For this review, take the finished solid that the model builds, in its own axes (mm). Face numbers are marked on the shaded views. A direction names the side the tool comes from. Round coordinates to 2 decimals unless told otherwise and drop trailing zeros. Order: outer loops, then holes, each group sorted by start corner. A loop starts at its lowest first (then second) coordinate and runs counter-clockwise, first axis right, second up.
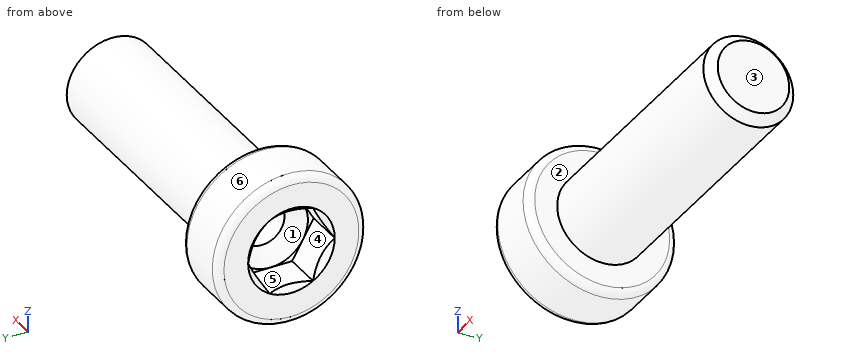
Autodesk Inventor part; units mm, degrees
ref_plane "MONTAGE_XY" through (0, 0, 0) normal (1, 0, 0) x (0, 0, -1)
ref_plane "MONTAGE_YZ" through (0, 0, 0) normal (0, 0, -1) x (0, 1, 0)
ref_plane "MONTAGE_ZX" through (0, 0, 0) normal (0, 1, 0) x (1, 0, 0)
sketch "Sketch_1" plane through (0, 0, 0) normal (0, 0, 1) x (1, 0, 0)
  line L0 (18, 0) -> (2.5, 0)
  line L1 (2.5, 0) -> (1, 1.5)
  line L2 (1, 1.5) -> (-0.5, 1.5)
  line L3 (-0.5, 1.5) -> (-1.5, 2.5)
  line L4 (-1.5, 2.5) -> (-3.6132, 2.5)
  line L5 (-3.6132, 2.5) -> (-4, 2.8868)
  line L6 (-4, 2.8868) -> (-4, 4.5)
  arc A0 (-3.5, 5) -> (-4, 4.5) centre (-3.5, 4.5) ccw
  line L7 (-3.5, 5) -> (-0.5, 5)
  arc A1 (0, 4.5) -> (-0.5, 5) centre (-0.5, 4.5) ccw
  line L8 (0, 4.5) -> (0, 3)
  line L9 (0, 3) -> (17.3865, 3)
  line L10 (17.3865, 3) -> (18, 2.3865)
  line L11 (18, 2.3865) -> (18, 0)
  line L12 (18, 0) -> (2.5, 0)
revolve "Revolution1" add sketch "Sketch_1" angle 360 about axis through (18, 0, 0) along (-1, 0, 0)
thread "Thread1"
sketch "Sketch_2" plane through (-4, 0, 0) normal (1, 0, 0) x (0, 0, -1)
  line L0 (-2.5, -1.4434) -> (0, -2.8868)
  line L1 (0, -2.8868) -> (2.5, -1.4434)
  line L2 (2.5, -1.4434) -> (2.5, 1.4434)
  line L3 (2.5, 1.4434) -> (0, 2.8868)
  line L4 (0, 2.8868) -> (-2.5, 1.4434)
  line L5 (-2.5, 1.4434) -> (-2.5, -1.4434)
extrude "Extrusion1" cut sketch "Sketch_2" along normal blind 2.5
ref_plane "MONTAGE_XY" through (0, 0, 0) normal (1, 0, 0) x (0, 0, -1)
ref_plane "MONTAGE_YZ" through (0, 0, 0) normal (0, 0, -1) x (0, 1, 0)
ref_plane "MONTAGE_ZX" through (0, 0, 0) normal (0, 1, 0) x (1, 0, 0)
ref_plane "Schrauben_punkt_XY" through (18, 0, 0) normal (-1, 0, 0) x (0, 0, -1)
ref_plane "Schrauben_punkt_YZ" through (18, 0, 0) normal (0, 0, -1) x (0, -1, 0)
ref_plane "Schrauben_punkt_ZX" through (18, 0, 0) normal (0, -1, 0) x (-1, 0, 0)
properties part number "DIN-6912 - M6x18(F)"
(1) Add section A-A on x = -2.25. Give the boundary of the cut face in (y, z), plus the area to 3 significant figures.
(2) Tool access review of the marked faces 1 and 2: name each direction out of +Z, -Z, +X, -X, +Y, -Y from which nothing blocks a thin tool from reaching the whole face with its end or side.
(3) Add section B-B on x = 9. Give the boundary of the cut face in (y, z), plus the area to 3 significant figures.
(4) Clearance check with flat-ended pins moving along their axes: P1, Ø6, axis at x = 15.5, y = 4, coming from the -Z side; P2, Ø1, axis at x = 5, y = 2.5, coming from the +Z side; P3, Ø0.7, axis at x = -3.5, y = -0.5, coming from the -Z side. State where each tip first meets the part, or that it passes through.
(5) Wall thickness on L1, parallel to Z at x = 0.7, y = 0; L2, parallel to X at y = -0.75, z = 0.75: over which ranges is each line inside the solid? List them lowest first.
(6) Draft analysis for pull direction Z (two halves, no side actions). For the marked faces 3, 4, 5 and 6, state which applies: pulls with the +Z half, pulls with the -Z half, needs draft (parallel to the pull), parting line crosses it, or undercut.
Here are the results:
1. outline: circle Ø10 at (0, 0); hole (-2.89, 0) - (-1.44, -2.5) - (1.44, -2.5) - (2.89, 0) - (1.44, 2.5) - (-1.44, 2.5) - close
1. area: 56.9 mm2
2. face 1: -X
2. face 2: +X
3. outline: circle Ø6 at (0, 0)
3. area: 28.3 mm2
4. P1: stops at z = -2.83
4. P2: stops at z = 2.24
4. P3: stops at z = -5
5. L1: z = -3 to -1.5, 1.5 to 3
5. L2: x = 1.44 to 18
6. face 3: needs draft
6. face 4: undercut
6. face 5: undercut
6. face 6: parting line crosses it
